Design review of the part built by this model. Coordinates are the model's own, in mm. Face numbers are marked on the shaded views. A direction names the side the tool comes from. Round coordinates to 2 decimals unless told otherwise and drop trailing zeros. Write each loop counter-clockwise with the first axis right and the second up, starting at its lowest first coordinate (ties: lowest second). Pieces come first, ordered by that corner, then holes. Notation, with made-up numbers: (38, 71.25) -> (73, 71.25) arc R27 ccw to (73, 89.25) -> close; hole circle Ø7 at (13, 30). An arc over 180 degrees is marked (long way). One line per question, with ' | ' between items. Start each with the question number.
1) Consider section A-A (x = 0). Give the boundary of the cut face in (y, z), then the cut area to 3 significant figures.
2) For probe 1 along Y at (x, z) = (0, 2.85); probe 2 along Y at (x, z) = (-0.5, 0); probe 3 along X at (y, z) = (97, 0), list the stretches that pass through material, from the lowest coordinate up.
3) Insertion check: pin 1 Ø1.5 at (x, z) = (-2.5, 3) entering from +Y; pin 2 Ø2 at (x, y) = (-2.5, 33.5) entering from +Z; pin 3 Ø3 at (y, z) = (81.5, 2) entering from +X; pin 4 Ø4 at (x, y) = (1.5, 21) entering from +Z. Each pin has a flat end and moves straight along its axis. Give the tip position at first contact, or say it passes through.
4) Consider section C-C (y = 59.5). Give the boundary of the cut face in (x, z), then the cut area to 3 significant figures.
5) For the marked faces 1 and 2, list the 3-axis set-ups (+Z, -Z, +X, -X, +Y, -Y) from which the entire face can be reached by the end or side of a thin tool; tool diameter is ignored.
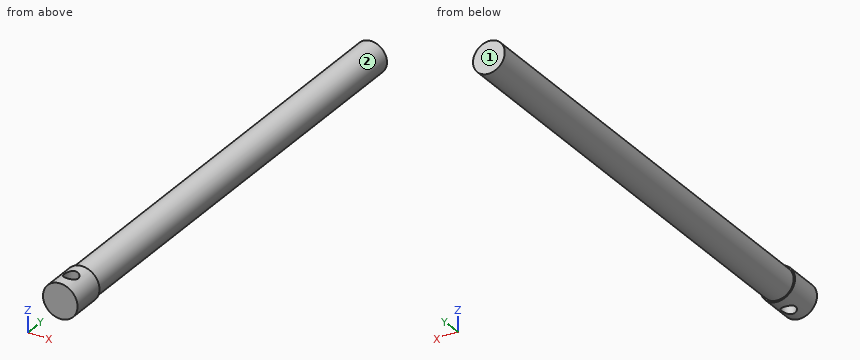
```python
from build123d import *

# Parameters (mm, degrees)
SKETCH1_R               = 3.937
BOSS_EXTRUDE1_DEPTH     = 7.9248
SKETCH3_R               = 3.6195
BOSS_EXTRUDE2_DEPTH     = 104.14
SKETCH4_R               = 1.5875
CUT_EXTRUDE1_DEPTH      = 4.937
CUT_EXTRUDE1_DEPTH_BACK = 4.937


with BuildPart() as part:
    # Sketch1 → Boss-Extrude1 (new body)
    with BuildSketch(Plane(origin=(0, 0, 0), x_dir=(1, 0, 0), z_dir=(0, 1, 0))):
        Circle(SKETCH1_R)
    extrude(amount=BOSS_EXTRUDE1_DEPTH)

    # Sketch3 → Boss-Extrude2 (add)
    with BuildSketch(Plane(origin=(0, 7.9248, 0), x_dir=(1, 0, 0), z_dir=(0, 1, 0))):
        Circle(SKETCH3_R)
    extrude(amount=BOSS_EXTRUDE2_DEPTH)

    # Sketch4 → Cut-Extrude1 (cut, two sides)
    with BuildSketch(Plane.XY) as cut_extrude1_sk:
        with Locations((0, 3.9624)):
            Circle(SKETCH4_R)
    extrude(amount=CUT_EXTRUDE1_DEPTH, mode=Mode.SUBTRACT)
    extrude(cut_extrude1_sk.sketch, amount=-CUT_EXTRUDE1_DEPTH_BACK, mode=Mode.SUBTRACT)


solid = part.part
```
From the geometry:
1) outline: (0, -3.94) -> (2.37, -3.94) -> (2.37, 3.94) -> (0, 3.94) -> close; (5.55, -3.94) -> (7.92, -3.94) -> (7.92, -3.62) -> (112.06, -3.62) -> (112.06, 3.62) -> (7.92, 3.62) -> (7.92, 3.94) -> (5.55, 3.94) -> close | area: 791 mm2
2) probe 1: y = 0 to 2.37, 5.55 to 112.06 | probe 2: y = 0 to 2.46, 5.47 to 112.06 | probe 3: x = -3.62 to 3.62
3) pin 1: stops at y = 112.06 | pin 2: stops at z = 3.29 | pin 3: stops at x = 3.58 | pin 4: stops at z = 3.62
4) outline: circle Ø7.24 at (0, 0) | area: 41.2 mm2
5) face 1: +Z, -Z, +X, -X, +Y | face 2: +Y
